from build123d import *

# Parameters (mm, degrees)
SKETCH008_W     = 20
SKETCH008_H     = 29
PAD008_DEPTH    = 15
PAD009_DEPTH    = 29
SKETCH017_R     = 4.75
PAD015_DEPTH    = 50
POCKET001_DEPTH = 70
SKETCH018_W     = 40
SKETCH018_H     = 15
POCKET002_DEPTH = 15
SKETCH019_R     = 5.05
POCKET003_DEPTH = 117
PAD016_DEPTH    = 20
SKETCH023_R     = 1.25
HOLE_DEPTH      = 25
HOLE_TIPS_R     = 1.25
SKETCH031_R     = 10.1
POCKET007_DEPTH = 30
SKETCH032_R     = 2.1
HOLE003_DEPTH   = 25
HOLE003_TIPS_R  = 2.1
CHAMFER001_SIZE = 1


with BuildPart() as part:
    # Sketch008 → Pad008 (new body)
    with BuildSketch(Plane.XY.offset(15)):
        with Locations((0, 35)):
            Rectangle(SKETCH008_W, SKETCH008_H)
        with BuildLine():
            ThreePointArc((-3, 39.5), (0, 29.591673), (3, 39.5))
            Line((3, 39.5), (3, 45.5))
            Line((3, 45.5), (-3, 45.5))
            Line((-3, 39.5), (-3, 45.5))
        make_face(mode=Mode.SUBTRACT)
    extrude(amount=PAD008_DEPTH)

    # Sketch009 → Pad009 (join)
    with BuildSketch(Plane.XZ.offset(-20.5)):
        with BuildLine():
            ThreePointArc((64.999803, -40), (0, 24.999803), (-64.999803, -40))
            Line((-64.999803, -40), (-40, -80))
            Line((-40, -80), (40, -80))
            Line((40, -80), (64.999803, -40))
        make_face()
    extrude(amount=-PAD009_DEPTH)

    # Sketch017 → Pad015 (join)
    with BuildSketch(Plane.XZ.offset(-10)):
        with Locations((0, -40)):
            Circle(SKETCH017_R)
    extrude(amount=-PAD015_DEPTH)

    # Sketch016 → Pocket001 (cut)
    with BuildSketch(Plane.XY.offset(30)):
        with BuildLine():
            ThreePointArc((-3, 39.5), (0, 29.591673), (3, 39.5))
            Line((3, 45.5), (3, 39.5))
            Line((-3, 45.5), (3, 45.5))
            Line((-3, 39.5), (-3, 45.5))
        make_face()
    extrude(amount=-POCKET001_DEPTH, mode=Mode.SUBTRACT)

    # Sketch018 → Pocket002 (cut)
    with BuildSketch(Plane.XZ.offset(-50)):
        with Locations((0, -22.5)):
            Rectangle(SKETCH018_W, SKETCH018_H)
    extrude(amount=POCKET002_DEPTH, mode=Mode.SUBTRACT)

    # Sketch019 → Pocket003 (cut)
    with BuildSketch(Plane.XZ):
        with Locations((-12.5, -22.5)):
            Circle(SKETCH019_R)
        with Locations((12.5, -22.5)):
            Circle(SKETCH019_R)
    extrude(amount=-POCKET003_DEPTH, mode=Mode.SUBTRACT)

    # Sketch022 → Pad016 (join)
    with BuildSketch(Plane.XZ.offset(-49.5)):
        Polygon((-10, -35), (-10, -30), (-20, -30), (-20, -15), (20, -15), (20, -30), (10, -30), (10, -35), (30, -35), (30, -20), (20, -10), (-20, -10), (-30, -20), (-30, -35), align=None)
    extrude(amount=-PAD016_DEPTH)

    # Sketch023 → Hole (cut)
    with BuildSketch(Plane.XZ.offset(-70)):
        with Locations((-25, -30)):
            Circle(SKETCH023_R)
        with Locations((25, -30)):
            Circle(SKETCH023_R)
        with Locations((-25, -22.5)):
            Circle(SKETCH023_R)
        with Locations((25, -22.5)):
            Circle(SKETCH023_R)
    extrude(amount=HOLE_DEPTH, mode=Mode.SUBTRACT)

    # Hole tips → Hole tip 1 section 0
    with BuildSketch(Plane.XZ.offset(-45), mode=Mode.PRIVATE) as hole_tip_1_s0:
        with Locations((-25, -30)):
            Circle(HOLE_TIPS_R)
    loft([hole_tip_1_s0.sketch, Vertex(-25, 44.248924, -30)], mode=Mode.SUBTRACT)

    # Hole tips → Hole tip 2 section 0
    with BuildSketch(Plane.XZ.offset(-45), mode=Mode.PRIVATE) as hole_tip_2_s0:
        with Locations((25, -30)):
            Circle(HOLE_TIPS_R)
    loft([hole_tip_2_s0.sketch, Vertex(25, 44.248924, -30)], mode=Mode.SUBTRACT)

    # Hole tips → Hole tip 3 section 0
    with BuildSketch(Plane.XZ.offset(-45), mode=Mode.PRIVATE) as hole_tip_3_s0:
        with Locations((-25, -22.5)):
            Circle(HOLE_TIPS_R)
    loft([hole_tip_3_s0.sketch, Vertex(-25, 44.248924, -22.5)], mode=Mode.SUBTRACT)

    # Hole tips → Hole tip 4 section 0
    with BuildSketch(Plane.XZ.offset(-45), mode=Mode.PRIVATE) as hole_tip_4_s0:
        with Locations((25, -22.5)):
            Circle(HOLE_TIPS_R)
    loft([hole_tip_4_s0.sketch, Vertex(25, 44.248924, -22.5)], mode=Mode.SUBTRACT)

    # Sketch031 → Pocket007 (cut)
    with BuildSketch(Plane.XZ.offset(-50)):
        with Locations((0, -60)):
            Circle(SKETCH031_R)
    extrude(amount=POCKET007_DEPTH, mode=Mode.SUBTRACT)

    # Sketch032 → Hole003 (cut)
    with BuildSketch(Plane.XZ.offset(-50)):
        with Locations((-15, -50)):
            Circle(SKETCH032_R)
        with Locations((-15, -70)):
            Circle(SKETCH032_R)
        with Locations((15, -70)):
            Circle(SKETCH032_R)
        with Locations((15, -50)):
            Circle(SKETCH032_R)
    extrude(amount=HOLE003_DEPTH, mode=Mode.SUBTRACT)

    # Hole003 tips → Hole003 tip 1 section 0
    with BuildSketch(Plane.XZ.offset(-25), mode=Mode.PRIVATE) as hole003_tip_1_s0:
        with Locations((-15, -50)):
            Circle(HOLE003_TIPS_R)
    loft([hole003_tip_1_s0.sketch, Vertex(-15, 23.738193, -50)], mode=Mode.SUBTRACT)

    # Hole003 tips → Hole003 tip 2 section 0
    with BuildSketch(Plane.XZ.offset(-25), mode=Mode.PRIVATE) as hole003_tip_2_s0:
        with Locations((-15, -70)):
            Circle(HOLE003_TIPS_R)
    loft([hole003_tip_2_s0.sketch, Vertex(-15, 23.738193, -70)], mode=Mode.SUBTRACT)

    # Hole003 tips → Hole003 tip 3 section 0
    with BuildSketch(Plane.XZ.offset(-25), mode=Mode.PRIVATE) as hole003_tip_3_s0:
        with Locations((15, -70)):
            Circle(HOLE003_TIPS_R)
    loft([hole003_tip_3_s0.sketch, Vertex(15, 23.738193, -70)], mode=Mode.SUBTRACT)

    # Hole003 tips → Hole003 tip 4 section 0
    with BuildSketch(Plane.XZ.offset(-25), mode=Mode.PRIVATE) as hole003_tip_4_s0:
        with Locations((15, -50)):
            Circle(HOLE003_TIPS_R)
    loft([hole003_tip_4_s0.sketch, Vertex(15, 23.738193, -50)], mode=Mode.SUBTRACT)

    # Chamfer001
    chamfer001_edges = [part.edges().sort_by_distance(p)[0] for p in [
        (3, 42.5, 30),
        (0, 45.5, 30),
        (-3, 42.5, 30),
        (0, 29.591673, 30),
        (-10, 35, 30),
        (0, 49.5, 30),
        (10, 35, 30),
        (0, 20.5, 30),
    ]]
    chamfer(chamfer001_edges, length=CHAMFER001_SIZE)


solid = part.part
Check sheet for the modelled part. Datum: model origin and axes. Units: mm. A direction names the side the tool comes from. Give positions to 0.01 mm unless a question says otherwise; leave off trailing zeros. Write each loop counter-clockwise with the first axis right and the second up, starting at its lowest first coordinate (ties: lowest second). Pieces come first, ordered by that corner, then holes. Notation, with made-up numbers: M 27,43.25 L 46,43.25 A15 ccw 46,50.25 Z; hole C 23,55 d2. An arc over 180 degrees is marked long. Use one line per item in the form item = value.
(1) Section check A-A on x = 0. State how many separate pieces and enclosed holes the cut face has, plus the area to 3 significant figures.
Answer block:
separate_pieces = 3
enclosed_holes = 0
area = 1,730 mm2
(2) Depth check by flat-ended pin: P1, Ø17.5, axis at x = 0.5, y = 56.5, coming from the -Z side; P2, Ø12, axis at x = 44.5, z = 14.5, coming from the -Y side; P3, Ø1.4, axis at y = 32.5, z = 26, coming from the +X side; P4, Ø5, axis at x = 50.5, z = -50, coming from the +Y side. Enter the tip coordinate at first touch or a pass-through.
Answer block:
P1 = -80
P2 = 20.5
P3 = 10
P4 = 49.5
(3) Tool access check on faces 1 (the flat face through (-20, 59, -35)), 2 (the flat face through (20, 52, -22)), 3 (the flat face through (3, 42, -35)), 4 (the flat face through (-10, 59, -33)), 5 (the cylindrical face through (-0.62, 15.18, -35.29)). Record the directions out of +Z, -Z, +X, -X, +Y, -Y that give a thin tool (end or side, any length) a straight path to the whole face; none if there is none.
Answer block:
face_1 = -Z, +X, -X, +Y
face_2 = +Y
face_3 = +Z
face_4 = -Z, +Y
face_5 = -Y
(4) Draft check along Z on faces 6 (the flat face through (52.325, 34.797, -60.28)), 7 (the cylindrical face through (-15.46, 37.42, -52.05)), 8 (the flat face through (10, 35, 27)). Enter one of: pulls with the +Z half, pulls with the -Z half, needs draft (parallel to the pull), parting line crosses it, or undercut.
Answer block:
face_6 = pulls with the -Z half
face_7 = undercut
face_8 = needs draft
(5) Section check D-D on x = 47.5. Record the boundary of the cut face in (y, z).
Answer block:
outline = M 20.5,-68 L 49.5,-68 L 49.5,4.37 L 20.5,4.37 Z
(6) Section check B-B on z = 5.5. Record the boundary of the cut face in (x, y), plus the area to 3 significant figures.
Answer block:
outline = M -46.42,20.5 L 46.42,20.5 L 46.42,49.5 L -46.42,49.5 Z; hole M -3,39.5 A5.41 ccw long 3,39.5 L 3,45.5 L -3,45.5 Z
area = 2,570 mm2
(7) Material ranges on line 1 along X through (y, z) = (58.75, -22.5); line 2 along Z through (x, y) = (-25, 54); line 3 along Z through (x, y) = (0, 30), recorded low to high.
Answer block:
line_1 = -30 to -26.25, -23.75 to -20, 20 to 23.75, 26.25 to 30
line_2 = -35 to -31.25, -28.75 to -23.75, -21.25 to -15
line_3 = -80 to -70.1, -49.9 to -40
